Here's the drawing with two shaded views (mm, measured from the low corner). I have some questions. Give positions to 0.01 mm unless a question says otherwise; leave off trailing zeros. Loops run counter-clockwise (first coordinate to the right, second up) from the corner with the lowest first, then second, coordinate; pieces in that order, holes last. Notation, with made-up numbers: (13.25, 70) -> (63.25, 70) arc R23 ccw to (63.25, 84) -> close; hole circle Ø8 at (74.25, 8.25). An arc over 180 degrees is marked (long way). Answer in a Markdown table with one row per item. Add a question column.
Item 1: If we section it at D-D (x = 9): Write out the boundary of the cut face in (y, z), then the cut area to 3 significant figures.
Item 2: If we section it at B-B (z = 54): Write out the boundary of the cut face in (x, y), then the cut area to 3 significant figures.
Item 3: If we section it at C-C (x = 58): Write out the boundary of the cut face in (y, z), then the cut area to 3 significant figures.
Item 4: For P1, Ø4, axis at x = 91.5, z = 77, coming from the -Y side; P2, Ø1.5, axis at x = 36, y = 1, coming from the -Z side; P3, Ø5, axis at y = 1, z = 46.5, coming from the +X side; P4, Ø6, axis at x = 54.5, y = 1, coming from the -Z side, each with a flat end and sliding along its axis, tell me the tip position at first contact or that it passes through.
Item 5: We'd pull the mould along Z, two halves only. Please class the marked faces 1, 2 and 3: released by +Z, released by -Z, zero draft, split by the parting line, or undercut.
Item 6: If I drill on line 1 (X direction, y = 6, z = 43); line 2 (X direction, y = 8.5, z = 58); line 3 (Z direction, x = 65.5, y = 8.5), over which ranges is the centre line in solid material (lowest first)?
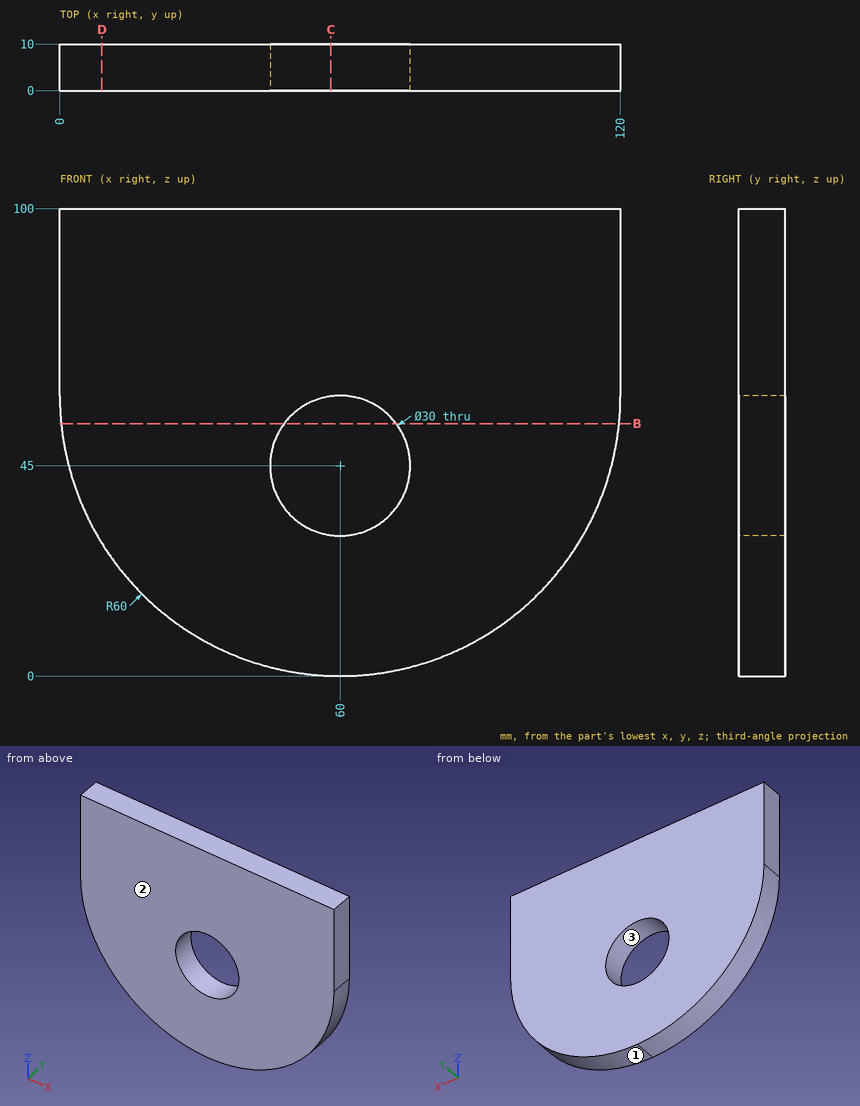
Recorded:
| question | item | result |
|---|---|---|
| 1 | outline | (0, 28.39) -> (10, 28.39) -> (10, 100) -> (0, 100) -> close |
| 1 | area | 716 mm^2 |
| 2 | outline | (0.3, 0) -> (48, 0) -> (48, 10) -> (0.3, 10) -> close; (72, 0) -> (119.7, 0) -> (119.7, 10) -> (72, 10) -> close |
| 2 | area | 954 mm^2 |
| 3 | outline | (0, 0.03) -> (10, 0.03) -> (10, 30.13) -> (0, 30.13) -> close; (0, 59.87) -> (10, 59.87) -> (10, 100) -> (0, 100) -> close |
| 3 | area | 702 mm^2 |
| 4 | P1 | stops at y = 0 |
| 4 | P2 | stops at z = 4.69 |
| 4 | P3 | stops at x = 118.98 |
| 4 | P4 | stops at z = 0.05 |
| 5 | face 1 | released by -Z |
| 5 | face 2 | zero draft |
| 5 | face 3 | undercut |
| 6 | line 1 | x = 2.46 to 45.13, 74.87 to 117.54 |
| 6 | line 2 | x = 0.03 to 52.52, 67.48 to 119.97 |
| 6 | line 3 | z = 0.25 to 31.04, 58.96 to 100 |
